For this review, use the dimensioned drawing (mm, ordinates from the lowest corner) and the shaded views. A direction names the side the tool comes from. Round coordinates to 2 decimals unless told otherwise and drop trailing zeros. Loops run counter-clockwise (first coordinate to the right, second up) from the corner with the lowest first, then second, coordinate; pieces in that order, holes last. Notation, with made-up numbers: M 75,0 L 115,0 A12 cw 115,12 Z; hole C -1,-6 d9. An arc over 180 degrees is marked long. Answer as a JSON object with one key per item and string values. Group by question number.
Item 1: Consider section D-D (x = 21.5). Give the boundary of the cut face in (y, z).
Item 2: Consider section A-A (x = 88.5). Give the boundary of the cut face in (y, z).
Item 3: To check wall thickness, follow line 1 (Y direction, x = 85, z = 10.5); line 2 (Z direction, x = 44.5, y = 67.5); line 3 (X direction, y = 57, z = 29). State the ranges of each line that lie inside material, in increasing order.
Item 4: The part is to be moulded in two halves that separate along Y. For the marked faces 4, 5 and 6, say which applies: +Y half, -Y half, draft (parallel to the pull), parting line (faces both ways), or undercut.
Item 5: Consider section B-B (y = 20.5). Give the boundary of the cut face in (x, z), and give its area (3 significant figures).
Item 6: Tool access review of the marked faces 1, 2 and 3: name each direction out of +Z, -Z, +X, -X, +Y, -Y from which nothing blocks a thin tool from reaching the whole face with its end or side.
Item 7: Consider section C-C (z = 13). Give the boundary of the cut face in (x, y), and give its area (3 significant figures).
Item 8: Insertion check: P1, Ø19, axis at x = 16.5, y = 42.5, coming from the +Z side; P2, Ø5, axis at y = 27, z = 29, coming from the +X side; P3, Ø4, axis at x = 92, y = 18, coming from the +Z side. Each pin has a flat end and moves straight along its axis. Give the tip position at first contact, or say it passes through.
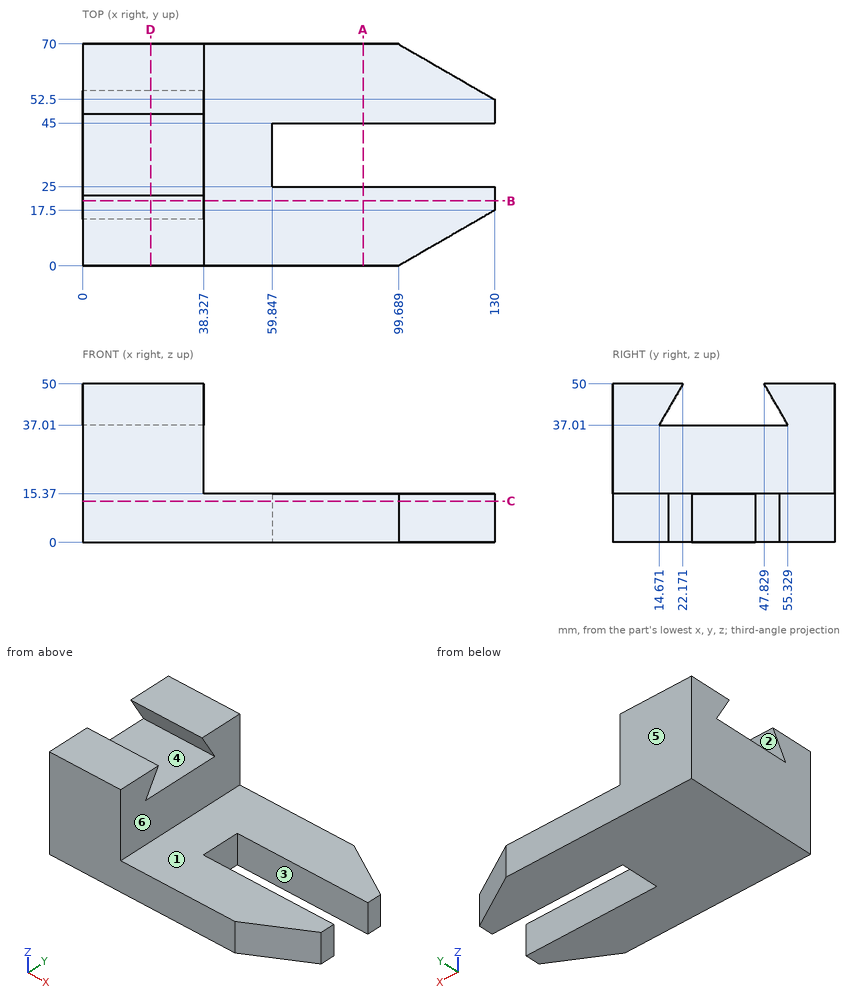
Geometry results:
{
 "1": {"outline": "M 0,0 L 70,0 L 70,50 L 47.83,50 L 55.33,37.01 L 14.67,37.01 L 22.17,50 L 0,50 Z"},
 "2": {"outline": "M 0,0 L 25,0 L 25,15.37 L 0,15.37 Z; M 45,0 L 70,0 L 70,15.37 L 45,15.37 Z"},
 "3": {"line 1": "y = 0 to 25, 45 to 70", "line 2": "z = 0 to 15.37", "line 3": "x = 0 to 38.33"},
 "4": {"face 4": "undercut", "face 5": "+Y half", "face 6": "draft"},
 "5": {"outline": "M 0,0 L 130,0 L 130,15.37 L 38.33,15.37 L 38.33,37.01 L 0,37.01 Z; M 0,47.11 L 38.33,47.11 L 38.33,50 L 0,50 Z", "area": "2,940 mm^2"},
 "6": {"face 1": "+Z, +X, +Y, -Y", "face 2": "+X, -X", "face 3": "+Z, -Z, +X"},
 "7": {"outline": "M 0,0 L 99.69,0 L 130,17.5 L 130,25 L 59.85,25 L 59.85,45 L 130,45 L 130,52.5 L 99.69,70 L 0,70 Z", "area": "7,170 mm^2"},
 "8": {"P1": "stops at z = 50", "P2": "stops at x = 38.33", "P3": "stops at z = 15.37"}
}
